Part model, mm, in its own coordinate system. Face numbers are marked on the shaded views. A direction names the side the tool comes from. Round coordinates to 2 decimals unless told otherwise and drop trailing zeros. Loops run counter-clockwise (first coordinate to the right, second up) from the corner with the lowest first, then second, coordinate; pieces in that order, holes last. Notation, with made-up numbers: M 64,39 L 111,39 A21 ccw 111,75 Z; hole C 61.25,14.25 d2. An arc over 180 degrees is marked long. Put each result on its own line as item: value. Start each with the question number.
1) Slice it at B-B on z = 2.25. Give the cut face in (x, y), then the cut area to 3 significant figures.
2) Probe line 1 along Y through (x, z) = (-6.5, 10.5); line 2 along X through (y, z) = (-3.75, 11); line 3 along Z through (x, y) = (-5.5, -24). List the from-to ranges inside material, lowest first.
3) Which spindle directions (+Z, -Z, +X, -X, +Y, -Y) get a long thin tool onto all of the face, cutting with end or side? Do the marked faces 1, 2, 3, 4 and 5. Say none if no direction does.
4) Drop flat-ended pins along their axis: pin 1 Ø10 at (x, z) = (12.5, 6) entering from -Y; pin 2 Ø3 at (y, z) = (-2.5, 3.5) entering from +X; pin 3 Ø3 at (x, y) = (5.5, -19.5) entering from +Z. Give the stop position or say it passes through.
5) Slice it at A-A on x = -2.5. Give the cut face in (y, z).
6) Slice it at C-C on y = -16.5. Give the cut face in (x, z).
```python
from build123d import *

# Parameters (mm, degrees)
F1_DEPTH = 6.35
F3_DEPTH = 25.4
F4_DEPTH = 25.4


with BuildPart() as f1:
    # F0 (on Front) → F1 (new body)
    with BuildSketch(Plane.XZ):
        Polygon((-25.4, 0), (0, 0), (25.4, 0), (25.4, 12.7), (-25.4, 12.7), align=None)
    extrude(amount=F1_DEPTH)

    # F2 (on Front) → F3 (join)
    with BuildSketch(Plane.XZ):
        Polygon((26.108526, -7.03671), (26.108526, 0), (0, 0), (-25.82779, 0), (-25.82779, -7.03671), align=None)
    extrude(amount=F3_DEPTH)

    # F2 (on Front) → F4 (join)
    with BuildSketch(Plane.XZ):
        Polygon((26.108526, -7.03671), (26.108526, 0), (0, 0), (-25.82779, 0), (-25.82779, -7.03671), align=None)
    extrude(amount=F4_DEPTH)


solid = f1.part
```
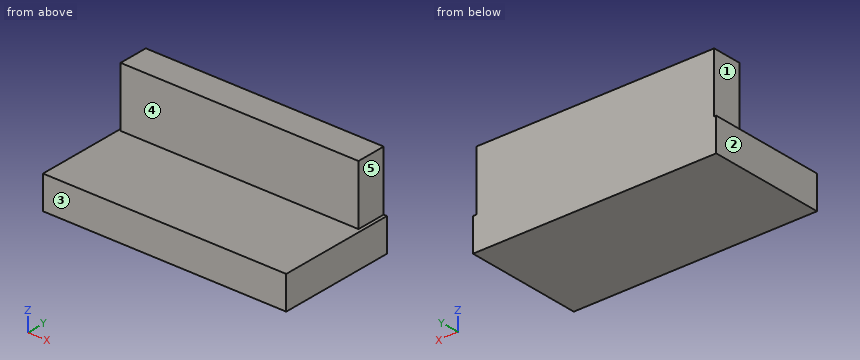
Recorded:
1. outline: M -25.4,-6.35 L 25.4,-6.35 L 25.4,0 L -25.4,0 Z
1. area: 323 mm2
2. line 1: y = -6.35 to 0
2. line 2: x = -25.4 to 25.4
2. line 3: z = -7.04 to 0
3. face 1: +Z, -X, +Y, -Y
3. face 2: +Z, -Z, -X, +Y, -Y
3. face 3: +Z, -Z, +X, -X, -Y
3. face 4: +Z, +X, -X, -Y
3. face 5: +Z, +X, +Y, -Y
4. pin 1: stops at y = -6.35
4. pin 2: stops at x = 25.4
4. pin 3: stops at z = 0
5. outline: M -25.4,-7.04 L 0,-7.04 L 0,12.7 L -6.35,12.7 L -6.35,0 L -25.4,0 Z
6. outline: M -25.83,-7.04 L 26.11,-7.04 L 26.11,0 L -25.83,0 Z
